Source: CAD feature listing. Evaluate the final solid. Frame: model axes, mm. Face numbers are marked on the shaded views. Give positions to 0.01 mm unless a question says otherwise; leave off trailing zeros. Loops run counter-clockwise (first coordinate to the right, second up) from the corner with the lowest first, then second, coordinate; pieces in that order, holes last. Notation, with made-up numbers: (-20, 82.25) - (-9, 82.25) arc R28 ccw to (-9, 121.25) - close; hole circle Ø8 at (4, 59.25). An arc over 180 degrees is marked (long way). Put each result on its own line as item: value.
```python
from build123d import *

# Parameters (mm, degrees)
SKETCH1_W               = 75
SKETCH1_H               = 20
BOSS_EXTRUDE1_DEPTH     = 4
CUT_EXTRUDE1_DEPTH      = 78.723870207
CUT_EXTRUDE1_DEPTH_BACK = 4
M2_CLEARANCE_HOLE1_D    = 2.4
CUT_EXTRUDE2_DEPTH      = 4


with BuildPart() as part:
    # Sketch1 → Boss-Extrude1 (new body)
    with BuildSketch(Plane(origin=(0, 0, 0), x_dir=(1, 0, 0), z_dir=(0, 1, 0))):
        with Locations((37.5, 10)):
            Rectangle(SKETCH1_W, SKETCH1_H)
    extrude(amount=BOSS_EXTRUDE1_DEPTH)

    # Sketch2 → Cut-Extrude1 (cut, two sides: drawn at the far end of the back side and taken through both)
    with BuildSketch(Plane(origin=(0, 4, 0), x_dir=(1, 0, 0), z_dir=(0, 1, 0)).offset(-CUT_EXTRUDE1_DEPTH_BACK)):
        with BuildLine():
            Line((0, 8.5), (10, 8.5))
            ThreePointArc((10, 8.5), (24.080201147, 10), (10, 11.5))
            Line((10, 11.5), (0, 11.5))
            Line((0, 11.5), (0, 10))
            Line((0, 10), (0, 8.5))
        make_face()
    extrude(amount=CUT_EXTRUDE1_DEPTH + CUT_EXTRUDE1_DEPTH_BACK, mode=Mode.SUBTRACT)

    # M2 Clearance Hole1 (through all)
    with Locations(Plane(origin=(0, 0, -20), x_dir=(-1, 0, 0), z_dir=(0, 0, -1))):
        with Locations((-4, 2)):
            Hole(M2_CLEARANCE_HOLE1_D / 2)

    # Sketch5 → Cut-Extrude2 (cut)
    with BuildSketch(Plane(origin=(0, 4, 0), x_dir=(1, 0, 0), z_dir=(0, 1, 0))):
        Polygon((0, 15.75), (7.691253114, 15.75), (11.941253114, 20), (0, 20), align=None)
        Polygon((0, 0), (0, 4.25), (7.691253114, 4.25), (11.941253114, 0), align=None)
    extrude(amount=-CUT_EXTRUDE2_DEPTH, mode=Mode.SUBTRACT)


solid = part.part
```
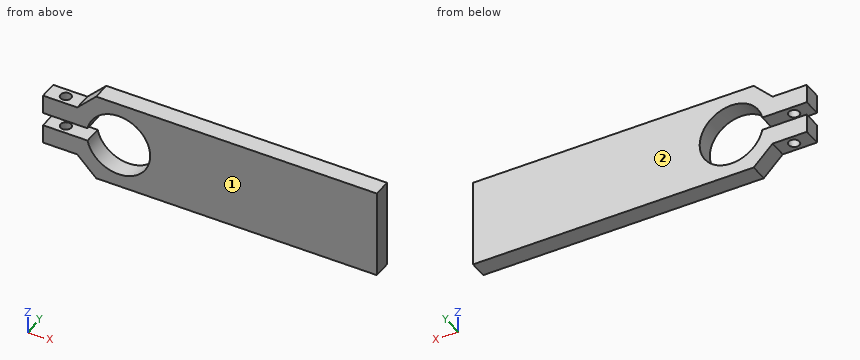
1) Mould query, pull axis Y, two halves, no side actions, for the marked faces 1 and 2. Classes: pulls with the +Y half, pulls with the -Y half, needs draft (parallel to the pull), parting line crosses it, or undercut.
Check result:
face 1: pulls with the -Y half
face 2: pulls with the +Y half
2) Material intervals for line 1 along Y through (x, z) = (4, -13.9); line 2 along X through (y, z) = (2.6, -6.25); line 3 along X through (y, z) = (1.5, -7.25), sorted ascending. Write a range as [from, to].
Check result:
line 1: [0, 0.8], [3.2, 4]
line 2: [0, 2.96], [5.04, 10.91], [23.01, 75]
line 3: [0, 2.91], [5.09, 10.39], [23.53, 75]
3) Pin query (flat end, axial travel): P1, Ø8.5, axis at x = 16.96, z = -10, coming from the +Y side. Return the tip coordinate at first contact, or that it passes through.
Check result:
P1: through
4) Section query B-B, the plane z = -7.5. Output: boundary loops of the cut face in (x, y), plus the area to 3 significant figures.
Check result:
outline: (0, 0) - (10.29, 0) - (10.29, 4) - (0, 4) - close; (23.63, 0) - (75, 0) - (75, 4) - (23.63, 4) - close; hole circle Ø2.4 at (4, 2)
area: 242 mm²
5) Section query A-A, the plane x = 6. Output: boundary loops of the cut face in (y, z), plus the area to 3 significant figures.
Check result:
outline: (0, -15.75) - (4, -15.75) - (4, -11.5) - (0, -11.5) - close; (0, -8.5) - (4, -8.5) - (4, -4.25) - (0, -4.25) - close
area: 34.0 mm²
6) Section query C-C, the plane x = 19.5. Output: boundary loops of the cut face in (y, z), plus the area to 3 significant figures.
Check result:
outline: (0, -20) - (4, -20) - (4, -16.65) - (0, -16.65) - close; (0, -3.35) - (4, -3.35) - (4, 0) - (0, 0) - close
area: 26.8 mm²
